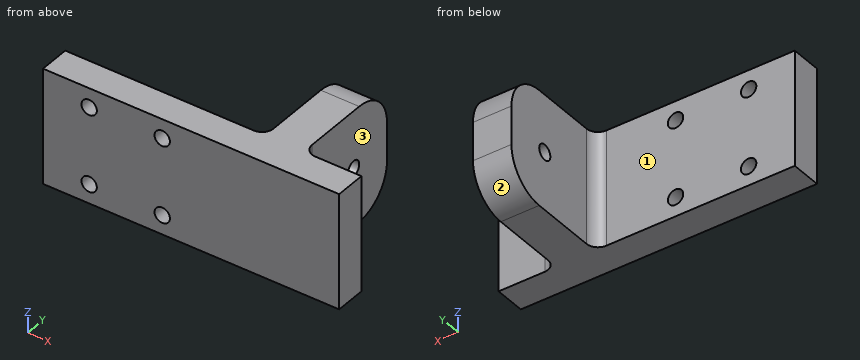
```python
from build123d import *

# Parameters (mm, degrees)
SKETCH1_W           = 40
SKETCH1_H           = 30
BOSS_EXTRUDE1_DEPTH = 8
SKETCH2_W           = 10
SKETCH2_H           = 30
BOSS_EXTRUDE2_DEPTH = 30
FILLET2_R           = 3
SKETCH4_R           = 2
CUT_EXTRUDE2_DEPTH  = 10
FILLET3_R           = 10
SKETCH5_W           = 30
SKETCH5_H           = 8
BOSS_EXTRUDE3_DEPTH = 37
SKETCH8_R           = 2
CUT_EXTRUDE3_DEPTH  = 37


with BuildPart() as part:
    # Sketch1 → Boss-Extrude1 (new body)
    with BuildSketch(Plane(origin=(0, 0, 0), x_dir=(1, 0, 0), z_dir=(0, 1, 0))):
        Rectangle(SKETCH1_W, SKETCH1_H)
    extrude(amount=BOSS_EXTRUDE1_DEPTH)

    # Sketch2 → Boss-Extrude2 (add)
    with BuildSketch(Plane(origin=(0, 8, 0), x_dir=(1, 0, 0), z_dir=(0, 1, 0))):
        Rectangle(SKETCH2_W, SKETCH2_H)
    extrude(amount=BOSS_EXTRUDE2_DEPTH)

    # Fillet2
    fillet2_edges = [part.edges().sort_by_distance(p)[0] for p in [
        (5, 8, 0),
        (-5, 8, 0),
    ]]
    fillet(fillet2_edges, radius=FILLET2_R)

    # Sketch4 → Cut-Extrude2 (cut)
    with BuildSketch(Plane(origin=(5, 0, 0), x_dir=(0, 0, -1), z_dir=(1, 0, 0))):
        with Locations((0, 26)):
            Circle(SKETCH4_R)
    extrude(amount=-CUT_EXTRUDE2_DEPTH, mode=Mode.SUBTRACT)

    # Fillet3
    fillet3_edges = [part.edges().sort_by_distance(p)[0] for p in [
        (0, 38, -15),
        (0, 38, 15),
    ]]
    fillet(fillet3_edges, radius=FILLET3_R)

    # Sketch5 → Boss-Extrude3 (add)
    with BuildSketch(Plane.ZY.offset(20)):
        with Locations((0, 4)):
            Rectangle(SKETCH5_W, SKETCH5_H)
    extrude(amount=BOSS_EXTRUDE3_DEPTH)

    # Sketch8 → Cut-Extrude3 (cut)
    with BuildSketch(Plane(origin=(0, 8, 0), x_dir=(1, 0, 0), z_dir=(0, 1, 0))):
        with Locations(Location((-45, 10, 0), (0, 0, 270))):
            Circle(SKETCH8_R)
        with Locations(Location((-45, -10, 0), (0, 0, 270))):
            Circle(SKETCH8_R)
        with Locations(Location((-26, -10, 0), (0, 0, 270))):
            Circle(SKETCH8_R)
        with Locations(Location((-26, 10, 0), (0, 0, 270))):
            Circle(SKETCH8_R)
    extrude(amount=-CUT_EXTRUDE3_DEPTH, mode=Mode.SUBTRACT)


solid = part.part
```
The listing builds one solid part. Answer for the finished solid, in the listing's coordinates (mm). Face numbers are marked on the shaded views. A direction names the side the tool comes from. Round coordinates to 2 decimals unless told otherwise and drop trailing zeros. Order: outer loops, then holes, each group sorted by start corner. A loop starts at its lowest first (then second) coordinate and runs counter-clockwise, first axis right, second up. Notation, with made-up numbers: (5, 54) -> (39, 54) arc R23 ccw to (39, 76) -> close; hole circle Ø8 at (-16.5, 22). An arc over 180 degrees is marked (long way). Answer as CSV lines item,"result". Start each with the question number.
(1) The part is cut by section A-A (x = -45). Determine the outline of the cut face in (y, z), then the cut area to 3 significant figures.
(2) A tool of negligible diameter and unlimited length cuts with its end or side. For the marked faces 1, 2 and 3, from which of +Z, -Z, +X, -X, +Y, -Y can it reach the whole face along a straight path? Write none if from no direction.
(3) The part is cut by section B-B (z = 0). Determine the outline of the cut face in (x, y).
(4) The part is cut by section D-D (y = 20). Determine the outline of the cut face in (x, z), then the cut area to 3 significant figures.
(5) Flat-ended cylindrical pins translate along their axes: pin 1 Ø13.5 at (y, z) = (23, -1) entering from +X; pin 2 Ø3 at (x, z) = (-17.5, 0) entering from +Y; pin 3 Ø13.5 at (y, z) = (19.5, 1.5) entering from -X; pin 4 Ø2.5 at (x, z) = (-26, -10) entering from +Y. Find the tip coordinate at first contact, or state that the pin passes through.
(6) Find the intervals of material crossed by probe 1 along X at (y, z) = (2.5, 10); probe 2 along Y at (x, z) = (10, -11); probe 3 along X at (y, z) = (17.5, 5.5), in increasing order. Write a range as from..to.
(7) The part is cut by section C-C (z = 9). Determine the outline of the cut face in (x, y).
Evaluation:
1,outline,"(0, -15) -> (8, -15) -> (8, -12) -> (0, -12) -> close; (0, -8) -> (8, -8) -> (8, 8) -> (0, 8) -> close; (0, 12) -> (8, 12) -> (8, 15) -> (0, 15) -> close"
1,area,"176 mm²"
2,face 1,"+Z, -Z, -X, +Y"
2,face 2,"-Z, +X, -X, +Y"
2,face 3,"+Z, -Z, +X, +Y"
3,outline,"(-57, 0) -> (20, 0) -> (20, 8) -> (8, 8) arc R3 cw to (5, 11) -> (5, 24) -> (-5, 24) -> (-5, 11) arc R3 cw to (-8, 8) -> (-57, 8) -> close; (-5, 28) -> (5, 28) -> (5, 38) -> (-5, 38) -> close"
4,outline,"(-5, -15) -> (5, -15) -> (5, 15) -> (-5, 15) -> close"
4,area,"300 mm²"
5,pin 1,"x = 5"
5,pin 2,"y = 8"
5,pin 3,"x = -5"
5,pin 4,"through"
6,probe 1,"-57..-47, -43..-28, -24..20"
6,probe 2,"0..8"
6,probe 3,"-5..5"
7,outline,"(-57, 0) -> (-46.73, 0) -> (-46.73, 8) -> (-57, 8) -> close; (-43.27, 0) -> (-27.73, 0) -> (-27.73, 8) -> (-43.27, 8) -> close; (-24.27, 0) -> (20, 0) -> (20, 8) -> (8, 8) arc R3 cw to (5, 11) -> (5, 37.17) -> (-5, 37.17) -> (-5, 11) arc R3 cw to (-8, 8) -> (-24.27, 8) -> close"
